Check sheet for the modelled part. Datum: model origin and axes. Units: mm. A direction names the side the tool comes from. Round coordinates to 2 decimals unless told otherwise and drop trailing zeros. Order: outer loops, then holes, each group sorted by start corner. A loop starts at its lowest first (then second) coordinate and runs counter-clockwise, first axis right, second up. Notation, with made-up numbers: (55, -31.75) -> (79, -31.75) arc R20 ccw to (79, -19.75) -> close; hole circle Ø8 at (27.5, 81.25). An arc over 180 degrees is marked (long way). Answer in a Markdown table with one row per item.
Autodesk Inventor part; units mm, degrees
ref_plane "YZ Plane" through (0, 0, 0) normal (1, 0, 0) x (0, 1, 0)
ref_plane "XZ Plane" through (0, 0, 0) normal (0, 1, 0) x (-1, 0, 0)
ref_plane "XY Plane" through (0, 0, 0) normal (0, 0, 1) x (1, 0, 0)
sketch "Sketch1" plane through (0, 0, 0) normal (1, 0, 0) x (0, 1, 0)
  line L0 (33.7, 0) -> (276.7, 0)
  line L1 (283.4, -6.7) -> (283.4, -60)
  line L2 (283.4, -60) -> (0, -60)
  line L3 (0, -60) -> (0, -6.7)
  line L4 (276.7, 0) -> (276.7, -6.7)
  line L5 (276.7, -6.7) -> (283.4, -6.7)
  line L6 (33.7, 0) -> (33.7, -6.7)
  line L7 (33.7, -6.7) -> (0, -6.7)
  point P0 (0, 0)
  dimension "d0" = 283.4
  dimension "d2" = 6.7
  dimension "d3" = 6.7
  dimension "d4" = 33.7
  dimension "d5" = 6.7
extrude "Extrusion1" add sketch "Sketch1" along normal blind 6.7
sketch "Sketch2" plane through (6.7, 0, 0) normal (1, 0, 0) x (0, 0, -1)
  line L0 (6.7, 276.7) -> (0, 276.7)
  line L1 (0, 276.7) -> (0, 249.7)
  line L2 (0, 276.7) -> (0, 33.7)
  line L3 (0, 249.7) -> (6.7, 249.7)
  line L4 (6.7, 249.7) -> (6.7, 222.7)
  line L5 (6.7, 222.7) -> (0, 222.7)
  line L6 (0, 222.7) -> (0, 249.7)
  point P0 (0, 0)
  dimension "d8" = 27
  dimension "d9" = 6.7
  dimension "d10" = 27
extrude "Extrusion2" cut sketch "Sketch2" against normal blind 6.7
pattern_linear "Rectangular Pattern1" count 4 spacing 54 along (0, -1, 0) of "Extrusion2"
sketch "Sketch3" plane through (6.7, 0, 0) normal (1, 0, 0) x (0, 0, -1)
  line L0 (60, 0) -> (60, 283.4)
  line L1 (60, 283.4) -> (40, 283.4)
  line L2 (40, 283.4) -> (40, 276.7)
  line L3 (40, 276.7) -> (60, 276.7)
  line L4 (60, 276.7) -> (60, 283.4)
  line L5 (60, 0) -> (40, 0)
  line L6 (40, 0) -> (40, 6.7)
  line L7 (40, 6.7) -> (60, 6.7)
  line L8 (60, 6.7) -> (60, 0)
  point P0 (0, 0)
  dimension "d16" = 20
  dimension "d17" = 20
  dimension "d18" = 6.7
  dimension "d19" = 6.7
extrude "Extrusion3" cut sketch "Sketch3" against normal blind 6.7
properties part number "b_base_support 2"
(1) Draft check along Y on faces 6 (the flat face through (3, 33.7, -3)), 7 (the flat face through (3, 74, -6.7)), 8 (the flat face through (3, 144, -60)). Enter one of: pulls with the +Y half, pulls with the -Y half, needs draft (parallel to the pull), parting line crosses it, or undercut.
Solutions:
| item | result |
|---|---|
| face 6 | pulls with the -Y half |
| face 7 | undercut |
| face 8 | needs draft |
(2) Tool access check on faces 1 (the flat face through (6.7, 140, -30)), 2 (the flat face through (3, 280, -6.7)), 3 (the flat face through (3, 168.7, -3)), 4 (the flat face through (3, 276.7, -50)), 5 (the flat face through (3, 209, 0)). Record the directions out of +Z, -Z, +X, -X, +Y, -Y that give a thin tool (end or side, any length) a straight path to the whole face; none if there is none.
Solutions:
| item | result |
|---|---|
| face 1 | +Z, -Z, +X, +Y, -Y |
| face 2 | +Z, +X, -X, +Y |
| face 3 | +Z, +X, -X |
| face 4 | -Z, +X, -X, +Y |
| face 5 | +Z, +X, -X, +Y, -Y |
(3) Depth check by flat-ended pin: pin 1 Ø3 at (x, z) = (3, -8.5) entering from -Y; pin 2 Ø2 at (x, y) = (4, 242.5) entering from +Z; pin 3 Ø2 at (x, z) = (2.5, -3) entering from +Y; pin 4 Ø3.5 at (x, z) = (4, -2.5) entering from -Y. Enter the tip coordinate at first touch or a pass-through.
Solutions:
| item | result |
|---|---|
| pin 1 | y = 0 |
| pin 2 | z = -6.7 |
| pin 3 | y = 276.7 |
| pin 4 | y = 33.7 |
(4) Section check A-A on x = 3.5. Record the boundary of the cut face in (y, z), plus the area to 3 significant figures.
Solutions:
| item | result |
|---|---|
| outline | (0, -40) -> (6.7, -40) -> (6.7, -60) -> (276.7, -60) -> (276.7, -40) -> (283.4, -40) -> (283.4, -6.7) -> (276.7, -6.7) -> (276.7, 0) -> (249.7, 0) -> (249.7, -6.7) -> (222.7, -6.7) -> (222.7, 0) -> (195.7, 0) -> (195.7, -6.7) -> (168.7, -6.7) -> (168.7, 0) -> (141.7, 0) -> (141.7, -6.7) -> (114.7, -6.7) -> (114.7, 0) -> (87.7, 0) -> (87.7, -6.7) -> (60.7, -6.7) -> (60.7, 0) -> (33.7, 0) -> (33.7, -6.7) -> (0, -6.7) -> close |
| area | 15,700 mm^2 |
(5) Scan lines: probe 1 along Y at (x, z) = (1.5, -6.5); probe 2 along Y at (x, z) = (4, -44); probe 3 along Z at (x, y) = (1, 188.5). Record each from-to range of solid material in increasing order. Write a range as from..to.
Solutions:
| item | result |
|---|---|
| probe 1 | 33.7..60.7, 87.7..114.7, 141.7..168.7, 195.7..222.7, 249.7..276.7 |
| probe 2 | 6.7..276.7 |
| probe 3 | -60..-6.7 |
(6) Section check C-C on y = 182.5. Record the boundary of the cut face in (x, z), plus the area to 3 significant figures.
Solutions:
| item | result |
|---|---|
| outline | (0, -60) -> (6.7, -60) -> (6.7, -6.7) -> (0, -6.7) -> close |
| area | 357 mm^2 |
(7) Section check B-B on z = -49. Record the boundary of the cut face in (x, y).
Solutions:
| item | result |
|---|---|
| outline | (0, 6.7) -> (6.7, 6.7) -> (6.7, 276.7) -> (0, 276.7) -> close |
